```python
from build123d import *

# Parameters (mm, degrees)
SKETCH1_W                      = 400
SKETCH1_H                      = 400
BOSS_EXTRUDE1_DEPTH            = 3
HOLE1_D                        = 55
HOLE1_DEPTH                    = 100
M3_CLEARANCE_HOLE2_D           = 3.6
CUT_EXTRUDE2_START             = 32
CUT_EXTRUDE2_OUTLINE_W         = 400
CUT_EXTRUDE2_OUTLINE_H         = 400
CUT_EXTRUDE2_DEPTH             = 3
M3_CLEARANCE_HOLE3_D           = 3.6
M3_CLEARANCE_HOLE3_CSINK_D     = 3.65
M3_CLEARANCE_HOLE3_CSINK_ANGLE = 90


# Read off the part's stored shape, not the designer's step: Cut-Extrude2
with BuildPart() as part:
    # Sketch1 → Boss-Extrude1 (new body)
    with BuildSketch(Plane(origin=(0, 32, 0), x_dir=(1, 0, 0), z_dir=(0, 1, 0))):
        with Locations((0, -52.110233191)):
            Rectangle(SKETCH1_W, SKETCH1_H)
    extrude(amount=BOSS_EXTRUDE1_DEPTH)

    # Hole1
    with Locations(Plane(origin=(0, 35, 0), x_dir=(1, 0, 0), z_dir=(0, 1, 0))):
        with Locations((0, 0)):
            Hole(HOLE1_D / 2, depth=HOLE1_DEPTH)

    # M3 Clearance Hole2 (through all)
    with Locations(Plane(origin=(0, 32, 0), x_dir=(-1, 0, 0), z_dir=(0, -1, 0))):
        with Locations((-33.428580586, 19.3), (33.428580586, 19.3), (0, -38.6)):
            Hole(M3_CLEARANCE_HOLE2_D / 2)

    # Cut-Extrude2 outline → Cut-Extrude2 (cut)
    with BuildSketch(Plane(origin=(0, 0, 0), x_dir=(1, 0, 0), z_dir=(0, 1, 0)).offset(CUT_EXTRUDE2_START)):
        with Locations((0, -52.110233191)):
            Rectangle(CUT_EXTRUDE2_OUTLINE_W, CUT_EXTRUDE2_OUTLINE_H)
        with BuildLine():
            Line((-140, -145), (-140, -40))
            ThreePointArc((-140, -40), (-136.468645007, -28.651707986), (-127.121626837, -21.310900739))
            ThreePointArc((-127.121626837, -21.310900739), (-103.31209295, -4.731224861), (-90.065586424, 21.081749027))
            ThreePointArc((-90.065586424, 21.081749027), (4.310811973, 92.399496211), (91.63719038, 12.604576122))
            ThreePointArc((91.63719038, 12.604576122), (42.071647748, -134.927150215), (-105.413194935, -184.632023928))
            ThreePointArc((-105.413194935, -184.632023928), (-130.137416921, -171.300876436), (-140, -145))
        make_face(mode=Mode.SUBTRACT)
    extrude(amount=CUT_EXTRUDE2_DEPTH, mode=Mode.SUBTRACT)

    # M3 Clearance Hole3 (through all)
    with Locations(Plane(origin=(0, 35, 0), x_dir=(1, 0, 0), z_dir=(0, 1, 0))):
        with Locations((-64.951905284, 37.5), (0, -75), (64.951905284, 37.5)):
            CounterSinkHole(M3_CLEARANCE_HOLE3_D / 2, M3_CLEARANCE_HOLE3_CSINK_D / 2, counter_sink_angle=M3_CLEARANCE_HOLE3_CSINK_ANGLE)


solid = part.part
```
The listing builds one solid part. Answer for the finished solid, in the listing's coordinates (mm). Round coordinates to 2 decimals unless told otherwise and drop trailing zeros. Write each loop counter-clockwise with the first axis right and the second up, starting at its lowest first coordinate (ties: lowest second). Pieces come first, ordered by that corner, then holes. Notation, with made-up numbers: (-4.75, -3) -> (19.25, -3) arc R30 ccw to (19.25, 23) -> close; hole circle Ø5 at (16, 52.25). An arc over 180 degrees is marked (long way). Use CSV: the item, a comma, the result in double quotes. Start each with the question number.
(1) Section B-B on z = 8 is taken. Give the vertices of the cut face in (x, y), then the cut area to 3 significant figures.
(2) This flat-tipped pin is pushed along its axis until it touches: pin 1 (1.5 mm diameter, centred on x = 64, y = 33, fed in from -Z). Where does it stop, or does it pass through?
(3) Section D-D on z = 47 is taken. Give the vertices of the cut face in (x, y), then the cut area to 3 significant figures.
(4) Section A-A on y = 32.75 is taken. Give the vertices of the cut face in (x, z), then the cut area to 3 significant figures.
(5) Consider L1, parallel to Z at x = 0, y = 34.15; L2, parallel to Z at x = 14, y = 33.15; L3, parallel to Z at x = 17, y = 32.95. Determine where each line is inside the solid, lowest interval first. Write a range as from..to.
(6) The mould has two halves that part along Z. Classify faces 1 (the face through (-129.872, 33.479, 171.602)), 2 (the face through (-103.583, 33.479, 5.039)), 3 (the face through (-25, 35, 45)), 4 (the face through (5.961, 33.479, 26.846)): released by +Z, released by -Z, zero draft, split by the parting line, or undercut.
(7) Section C-C on z = -61.5 is taken. Give the vertices of the cut face in (x, y), then the cut area to 3 significant figures.
A:
1,outline,"(-106.39, 32) -> (-26.31, 32) -> (-26.31, 35) -> (-106.39, 35) -> close; (26.31, 32) -> (93.24, 32) -> (93.24, 35) -> (26.31, 35) -> close"
1,area,"441 mm²"
2,pin 1,"stops at z = -67.5"
3,outline,"(-140, 32) -> (89.58, 32) -> (89.58, 35) -> (-140, 35) -> close"
3,area,"689 mm²"
4,outline,"(-140, 40) arc R20 ccw to (-127.12, 21.31) arc R60 cw to (-90.07, -21.08) arc R92.5 ccw to (91.64, -12.6) arc R175 ccw to (-105.41, 184.63) arc R40 ccw to (-140, 145) -> close; hole circle Ø3.6 at (-64.95, -37.5); hole circle Ø3.6 at (-33.43, -19.3); hole circle Ø55 at (0, 0); hole circle Ø3.6 at (0, 38.6); hole circle Ø3.6 at (0, 75); hole circle Ø3.6 at (33.43, -19.3); hole circle Ø3.6 at (64.95, -37.5)"
4,area,"46,800 mm²"
5,L1,"z = -92.5..-27.5, 27.5..36.8, 40.4..73.2, 76.8..165.98"
5,L2,"z = -91.43..-23.67, 23.67..157.74"
5,L3,"z = -90.92..-21.62, 21.62..155.73"
6,face 1,"released by +Z"
6,face 2,"released by -Z"
6,face 3,"zero draft"
6,face 4,"undercut"
7,outline,"(-69.09, 32) -> (69.09, 32) -> (69.09, 35) -> (-69.09, 35) -> close"
7,area,"415 mm²"
